```python
from build123d import *

# Parameters (mm, degrees)
SZKIC1_W                    = 70
SZKIC1_H                    = 32
DODANIE_WYCI_GNI_CIE1_DEPTH = 10
SZKIC2_W                    = 10
SZKIC2_H                    = 32
DODANIE_WYCI_GNI_CIE2_DEPTH = 20
SZKIC3_W                    = 70
SZKIC3_H                    = 12
DODANIE_WYCI_GNI_CIE3_DEPTH = 26
SZKIC4_W                    = 70
SZKIC4_H                    = 6
DODANIE_WYCI_GNI_CIE4_DEPTH = 20
SZKIC5_R                    = 0.5
WYTNIJ_WYCI_GNI_CIE1_DEPTH  = 83.607505712
ZAOKR_GLENIE1_R             = 2
SZKIC6_R                    = 8
WYTNIJ_WYCI_GNI_CIE2_DEPTH  = 83.607505712
ZAOKR_GLENIE2_R             = 10
SZKIC7_R                    = 2.6
WYTNIJ_WYCI_GNI_CIE3_DEPTH  = 79.74007874
SZKIC8_R                    = 2.6
WYTNIJ_WYCI_GNI_CIE4_DEPTH  = 20
SFAZOWANIE1_SIZE            = 6


with BuildPart() as part:
    # Szkic1 → Dodanie-wyciągnięcie1 (new body)
    with BuildSketch(Plane.XY):
        with Locations((35, 16)):
            Rectangle(SZKIC1_W, SZKIC1_H)
    extrude(amount=DODANIE_WYCI_GNI_CIE1_DEPTH)

    # Szkic2 → Dodanie-wyciągnięcie2 (add)
    with BuildSketch(Plane.XY.offset(10)):
        with Locations((5, 16)):
            Rectangle(SZKIC2_W, SZKIC2_H)
        with Locations((35, 16)):
            Rectangle(SZKIC2_W, SZKIC2_H)
        with Locations((65, 16)):
            Rectangle(SZKIC2_W, SZKIC2_H)
    extrude(amount=DODANIE_WYCI_GNI_CIE2_DEPTH)

    # Szkic3 → Dodanie-wyciągnięcie3 (add)
    with BuildSketch(Plane(origin=(0, 0, 0), x_dir=(-1, 0, 0), z_dir=(0, 0, -1))):
        with Locations((-35, 26)):
            Rectangle(SZKIC3_W, SZKIC3_H)
    extrude(amount=DODANIE_WYCI_GNI_CIE3_DEPTH)

    # Szkic4 → Dodanie-wyciągnięcie4 (add)
    with BuildSketch(Plane.XZ.offset(-20)):
        with Locations((35, -23)):
            Rectangle(SZKIC4_W, SZKIC4_H)
    extrude(amount=DODANIE_WYCI_GNI_CIE4_DEPTH)

    # Szkic5 → Wytnij-wyciągnięcie1 (cut, through all)
    with BuildSketch(Plane.ZY):
        with Locations((-20, 20)):
            Circle(SZKIC5_R)
        with Locations((0, 20)):
            Circle(SZKIC5_R)
    extrude(amount=-WYTNIJ_WYCI_GNI_CIE1_DEPTH, mode=Mode.SUBTRACT)

    # Zaokrąglenie1
    zaokr_glenie1_edges = [part.edges().sort_by_distance(p)[0] for p in [
        (35, 19.5, -20),
        (35, 19.5, 0),
        (35, 20, -19.5),
        (35, 20, -0.5),
    ]]
    fillet(zaokr_glenie1_edges, radius=ZAOKR_GLENIE1_R)

    # Szkic6 → Wytnij-wyciągnięcie2 (cut, through all)
    with BuildSketch(Plane.ZY):
        with Locations((20, 16)):
            Circle(SZKIC6_R)
    extrude(amount=-WYTNIJ_WYCI_GNI_CIE2_DEPTH, mode=Mode.SUBTRACT)

    # Zaokrąglenie2
    zaokr_glenie2_edges = [part.edges().sort_by_distance(p)[0] for p in [
        (5, 0, 30),
        (5, 32, 30),
        (35, 0, 30),
        (35, 32, 30),
        (65, 32, 30),
        (65, 0, 30),
    ]]
    fillet(zaokr_glenie2_edges, radius=ZAOKR_GLENIE2_R)

    # Szkic7 → Wytnij-wyciągnięcie3 (cut, through all)
    with BuildSketch(Plane.XZ.offset(-20)):
        with Locations(Location((20, -10, 0), (0, 0, 270))):
            Circle(SZKIC7_R)
        with Locations(Location((50, -10, 0), (0, 0, 270))):
            Circle(SZKIC7_R)
    extrude(amount=-WYTNIJ_WYCI_GNI_CIE3_DEPTH, mode=Mode.SUBTRACT)

    # Szkic8 → Wytnij-wyciągnięcie4 (cut)
    with BuildSketch(Plane(origin=(0, 0, -26), x_dir=(-1, 0, 0), z_dir=(0, 0, -1))):
        with Locations((-35, 10)):
            Circle(SZKIC8_R)
    extrude(amount=-WYTNIJ_WYCI_GNI_CIE4_DEPTH, mode=Mode.SUBTRACT)

    # Sfazowanie1
    sfazowanie1_edges = [part.edges().sort_by_distance(p)[0] for p in [
        (35, 32, -26),
    ]]
    chamfer(sfazowanie1_edges, length=SFAZOWANIE1_SIZE)


solid = part.part
```
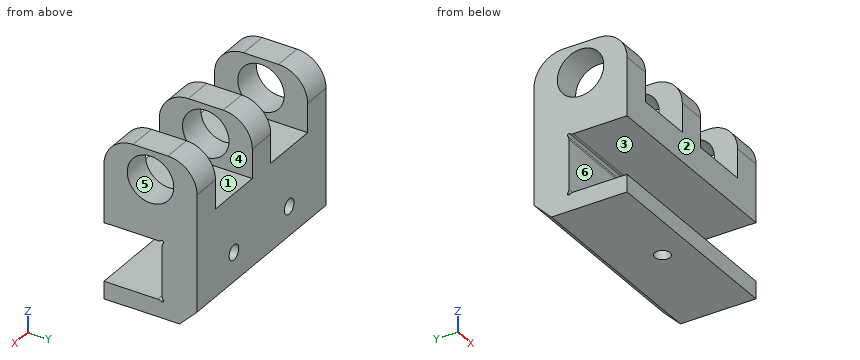
The listing builds one solid part. Answer for the finished solid, in the listing's coordinates (mm). Face numbers are marked on the shaded views. A direction names the side the tool comes from. Round coordinates to 2 decimals unless told otherwise and drop trailing zeros. Loops run counter-clockwise (first coordinate to the right, second up) from the corner with the lowest first, then second, coordinate; pieces in that order, holes last. Notation, with made-up numbers: (49.5, -1) - (71.5, -1) arc R24 cw to (71.5, 27) - close; hole circle Ø9 at (72.25, 63.5). An arc over 180 degrees is marked (long way). Use one line per item in the form item = value. Start each with the question number.
1. The part is cut by section B-B on z = 11. Determine the outline of the cut face in (x, y).
2. The part is cut by section A-A on x = 35. Determine the outline of the cut face in (y, z).
3. The part is cut by section C-C on y = 16. Determine the outline of the cut face in (x, z), then the cut area to 3 significant figures.
4. The part is cut by section D-D on x = 55. Determine the outline of the cut face in (y, z).
5. For a pull along Z with two mould halves and no side action, classify the marked faces 1, 2 and 3 as pulls with the +Z half, pulls with the -Z half, needs draft (parallel to the pull), parting line crosses it, or undercut.
6. Given pin 1 Ø8 at (x, z) = (37.5, 5.5) entering from -Y; pin 2 Ø4 at (x, y) = (16.5, 7.5) entering from +Z; pin 3 Ø8.5 at (x, z) = (36.5, -7.5) entering from -Y, each flat-ended and moving along its own axis, determine where each tip first touches the part or whether it passes through.
7. A tool of negligible diameter and unlimited length cuts with its end or side. For the marked faces 4, 5 and 6, from which of +Z, -Z, +X, -X, +Y, -Y can it reach the whole face along a straight path? Write none if from no direction.
8. Consider line 1 (X direction, y = 28.5, z = -10); line 2 (X direction, y = 19.5, z = 11.5); line 3 (Y direction, x = 35, z = -24). Determine where each line is inside the solid, lowest interval first. Write a range as [from, to].
Geometry check:
q1.outline = (0, 0) - (10, 0) - (10, 32) - (0, 32) - close; (30, 0) - (40, 0) - (40, 32) - (30, 32) - close; (60, 0) - (70, 0) - (70, 32) - (60, 32) - close
q2.outline = (0, -26) - (7.4, -26) - (7.4, -20) - (0, -20) - close; (0, 0) - (18.5, 0) arc R2 ccw to (19.7, 0.4) arc R0.5 cw to (20.4, -0.3) arc R2 ccw to (20, -1.5) - (20, -18.5) arc R2 ccw to (20.4, -19.7) arc R0.5 cw to (19.7, -20.4) arc R2 ccw to (18.5, -20) - (12.6, -20) - (12.6, -26) - (26, -26) - (32, -20) - (32, 20) arc R10 ccw to (22, 30) - (10, 30) arc R10 ccw to (0, 20) - close; hole circle Ø16 at (16, 20)
q3.outline = (0, -26) - (70, -26) - (70, -20) - (0, -20) - close; (0, 0) - (70, 0) - (70, 12) - (60, 12) - (60, 10) - (40, 10) - (40, 12) - (30, 12) - (30, 10) - (10, 10) - (10, 12) - (0, 12) - close; (0, 28) - (10, 28) - (10, 30) - (0, 30) - close; (30, 28) - (40, 28) - (40, 30) - (30, 30) - close; (60, 28) - (70, 28) - (70, 30) - (60, 30) - close
q3.area = 1,240 mm^2
q4.outline = (0, -26) - (26, -26) - (32, -20) - (32, 10) - (0, 10) - (0, 0) - (18.5, 0) arc R2 ccw to (19.7, 0.4) arc R0.5 cw to (20.4, -0.3) arc R2 ccw to (20, -1.5) - (20, -18.5) arc R2 ccw to (20.4, -19.7) arc R0.5 cw to (19.7, -20.4) arc R2 ccw to (18.5, -20) - (0, -20) - close
q5.face_1 = pulls with the +Z half
q5.face_2 = needs draft
q5.face_3 = undercut
q6.pin_1 = 0
q6.pin_2 = 10
q6.pin_3 = 20
q7.face_4 = +Z, +Y, -Y
q7.face_5 = +X, -X
q7.face_6 = +X, -X, -Y
q8.line_1 = [0, 17.4], [22.6, 47.4], [52.6, 70]
q8.line_2 = [0, 10], [30, 40], [60, 70]
q8.line_3 = [0, 7.4], [12.6, 28]
